from build123d import *

# Parameters (mm, degrees)
F0_W     = 75.2491950989
F0_H     = 48.5349902883
F1_DEPTH = 62.992
F2_ANGLE = 175
F3_ANGLE = -180


with BuildPart() as f1:
    # F0 (on Top) → F1 (new body)
    with BuildSketch(Plane.XY):
        with Locations((-3.7127323449, 11.5366871469)):
            Rectangle(F0_W, F0_H)
    extrude(amount=F1_DEPTH)


with BuildPart() as f1_1:
    # F2: moved
    add(f1.part.rotate(Axis((33.9118652046, 35.804182291, 31.496), (0, 0, -1)), F2_ANGLE))


with BuildPart() as f1_2:
    # F3: moved
    add(f1_1.part.rotate(Axis((31.7968136407, 59.9793322896, 0), (0.0871557427, -0.9961946981, 0)), F3_ANGLE))


solid = f1_2.part
The listing builds one solid part. Answer for the finished solid, in the listing's coordinates (mm). Coordinates: 2 decimals unless noted, no trailing zeros. Loops run counter-clockwise (first coordinate to the right, second up) from the corner with the lowest first, then second, coordinate; pieces in that order, holes last. Notation, with made-up numbers: (77.5, -39.75) -> (94.5, -39.75) arc R7 ccw to (94.5, -31.75) -> close; hole circle Ø3 at (83, -10.75). An arc over 180 degrees is marked (long way). Write item = value, one per line. Start each with the question number.
1) Given pin 1 Ø12 at (y, z) = (43, -38.5) entering from +X; pin 2 Ø8 at (y, z) = (52, -44.5) entering from -X; pin 3 Ø2 at (x, z) = (14, -14.5) entering from +Y, each flat-ended and moving along its own axis, determine where each tip first touches the part or whether it passes through.
2) Straight lines are drawn through the part: line 1 (X direction, y = 45.5, z = -50); line 2 (Y direction, x = 10, z = -23); line 3 (Y direction, x = 18, z = -29). For each, find the intervals that lie inside material, in ascending order. Write a range as from..to.
3) A cutting plane is placed at A-A (z = -15.5). Give the vertices of the cut face in (x, y), then the cut area to 3 significant figures.
4) A cutting plane is placed at B-B (y = 74). Give the vertices of the cut face in (x, z).
Responses:
q1.pin_1 = 33.81
q1.pin_2 = -43.39
q1.pin_3 = 82.87
q2.line_1 = -42.47..33.06
q2.line_2 = 33.71..82.43
q2.line_3 = 34.41..83.13
q3.outline = (-45.28, 77.6) -> (-41.05, 29.25) -> (33.91, 35.8) -> (29.68, 84.15) -> close
q3.area = 3,650 mm²
q4.outline = (-44.97, -62.99) -> (30.57, -62.99) -> (30.57, 0) -> (-44.97, 0) -> close
